CAD build for the part. Positions are in the model's coordinates, mm. Face numbers are marked on the shaded views. A direction names the side the tool comes from. Round coordinates to 2 decimals unless told otherwise and drop trailing zeros. Loops run counter-clockwise (first coordinate to the right, second up) from the corner with the lowest first, then second, coordinate; pieces in that order, holes last. Notation, with made-up numbers: M 74.5,1.5 L 129.5,1.5 A11 ccw 129.5,19.5 Z; hole C 54,-36 d7. An arc over 180 degrees is marked long. Use one line per item in the form item = value.
from build123d import *
from build123d import SkipClean  # not in build123d's __all__

# Parameters (mm, degrees)
F0_W     = 2.5400003581
F0_H     = 17.78
F0_H_2   = 2.54
F0_W_2   = 25.3999996419
F1_DEPTH = 152.4
F4_D     = 2.9464
F2_W     = 12.7
F2_H     = 21.717
F5_DEPTH = 2.54
F6_D     = 2.9464
F7_D     = 2.9464
F8_D     = 2.9464
F9_D     = 2.9464
F10_D    = 2.9464
F11_D    = 2.9464


# Not quite as in the source:
# - after a boolean that leaves OpenCascade's solid faulty, fix() repairs it
# - a feature names something its author has since deleted; it is built from what else it names


with BuildPart() as f1:
    # F0 (on Top) → F1 (new body)
    with BuildSketch(Plane.XY):
        with Locations((-9.334868336, -17.2625129279)):
            Rectangle(F0_W, F0_H)
        with Locations((-9.334868336, -7.1025129279)):
            Rectangle(F0_W, F0_H_2)
        with Locations((4.635131664, -7.1025129279)):
            Rectangle(F0_W_2, F0_H_2)
    extrude(amount=F1_DEPTH)

    # F4 (through all)
    with Locations(Plane(origin=(0, -5.8325129279, 0), x_dir=(-1, 0, 0), z_dir=(0, 1, 0))):
        with Locations((0.317868515, 78.1684368849)):
            Hole(F4_D / 2)

    # F2 (on face) → F5 (cut, symmetric)
    with BuildSketch(Plane(origin=(0, -5.8325129279, 0), x_dir=(-1, 0, 0), z_dir=(0, 1, 0))):
        with Locations((1.714868515, 114.0894710903)):
            Rectangle(F2_W, F2_H)
        with Locations((1.714868515, 92.3724710903)):
            Rectangle(F2_W, F2_H)
        with Locations((-10.985131485, 114.0894710903)):
            Rectangle(F2_W, F2_H)
        with Locations((-10.985131485, 92.3724710903)):
            Rectangle(F2_W, F2_H)
    with SkipClean():  # cleaning this boolean's faces spoils the solid; the shape is the same uncleaned
        extrude(amount=F5_DEPTH, both=True, mode=Mode.SUBTRACT)

    # F6 (through all)
    with Locations(Plane(origin=(0, -5.8325129279, 0), x_dir=(-1, 0, 0), z_dir=(0, 1, 0))):
        with Locations((0.317868515, 128.2935052958)):
            Hole(F6_D / 2)

    add(f1.part.fix(), mode=Mode.REPLACE)

    # F7 (through all)
    with Locations(Plane(origin=(0, -5.8325129279, 0), x_dir=(-1, 0, 0), z_dir=(0, 1, 0))):
        with Locations((-9.588131485, 128.2935052958)):
            Hole(F7_D / 2)

    # F8 (through all)
    with Locations(Plane(origin=(0, -5.8325129279, 0), x_dir=(-1, 0, 0), z_dir=(0, 1, 0))):
        with Locations((-9.588131485, 78.1684368849)):
            Hole(F8_D / 2)

    # F9 (through all)
    with Locations(Plane(origin=(0, -5.8325129279, 0), x_dir=(-1, 0, 0), z_dir=(0, 1, 0))):
        with Locations((-3.9381445386, 140.0028020144)):
            Hole(F9_D / 2)

    # F10 (through all)
    with Locations(Plane(origin=(0, -5.8325129279, 0), x_dir=(-1, 0, 0), z_dir=(0, 1, 0))):
        with Locations((-1.56237185, 24.8921643943)):
            Hole(F10_D / 2)

    # F11 (through all)
    with Locations(Plane(origin=(-10.604868515, 0, 0), x_dir=(0, -1, 0), z_dir=(-1, 0, 0))):
        with Locations((25.3072194755, 11.6721792147)):
            Hole(F11_D / 2)


solid = f1.part
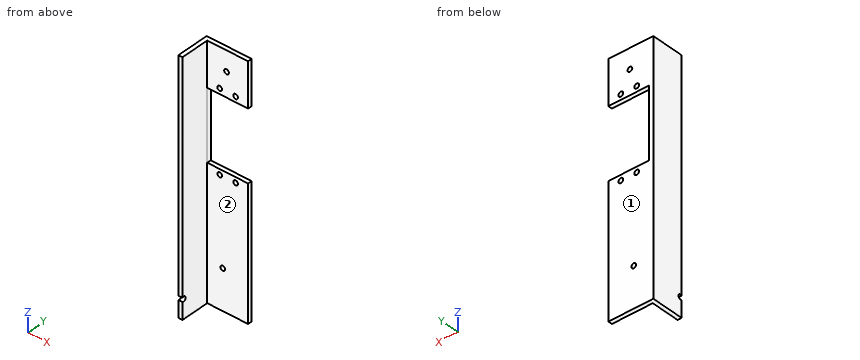
1. Cut at C-C on z = 30. Write the cut outline in (x, y), and give its area (3 significant figures).
Completed:
outline = M -10.6,-26.15 L -8.06,-26.15 L -8.06,-8.37 L 17.34,-8.37 L 17.34,-5.83 L -10.6,-5.83 Z
area = 116 mm2
2. Drop flat-ended pins along their axis: P1, Ø7.5, axis at x = 6, z = 32, coming from the -Y side; P2, Ø2, axis at y = -7.5, z = 94.5, coming from the +X side. Give the stop position or say it passes through.
Completed:
P1 = -8.37
P2 = -8.06
3. Cut at D-D on y = -22.25. Write the cut outline in (x, z), and give its area (3 significant figures).
Completed:
outline = M -10.6,0 L -8.06,0 L -8.06,152.4 L -10.6,152.4 Z
area = 387 mm2
4. Cut at B-B on x = -5.75. Write the cut outline in (y, z), and give its area (3 significant figures).
Completed:
outline = M -8.37,0 L -5.83,0 L -5.83,81.51 L -8.37,81.51 Z; M -8.37,124.95 L -5.83,124.95 L -5.83,152.4 L -8.37,152.4 Z
area = 277 mm2
5. Cut at A-A on x = 9.5. Write the cut outline in (y, z), and give its area (3 significant figures).
Completed:
outline = M -8.37,0 L -5.83,0 L -5.83,76.7 L -8.37,76.7 Z; M -8.37,79.64 L -5.83,79.64 L -5.83,81.51 L -8.37,81.51 Z; M -8.37,124.95 L -5.83,124.95 L -5.83,126.82 L -8.37,126.82 Z; M -8.37,129.76 L -5.83,129.76 L -5.83,152.4 L -8.37,152.4 Z
area = 262 mm2
6. Probe line 1 along X through (y, z) = (-20.5, 99); line 2 along Y through (x, z) = (5.25, 67); line 3 along Z through (x, y) = (-1, -7). List the from-to ranges inside material, lowest first. Write a range as from..to.
Completed:
line_1 = -10.6..-8.06
line_2 = -8.37..-5.83
line_3 = 0..76.86, 79.47..81.51, 124.95..126.99, 129.6..152.4
7. Tool access for the marked faces 1 and 2: list every direction of +Z, -Z, +X, -X, +Y, -Y with a clear straight run to the whole face (end or side of a thin tool).
Completed:
face_1 = +Z, -Z, +X, -X, +Y
face_2 = +Z, -Z, +X, -Y
